Geometry: final body of the model. Coordinates: model frame, mm. Give positions to 0.01 mm unless a question says otherwise; leave off trailing zeros. Order: outer loops, then holes, each group sorted by start corner. A loop starts at its lowest first (then second) coordinate and runs counter-clockwise, first axis right, second up. Notation, with made-up numbers: (-28, 49.5) - (10, 49.5) arc R6 ccw to (10, 59.5) - close; hole circle Ø7 at (-13.5, 70). An arc over 180 degrees is marked (long way). One line per question, with ' | ' between items. Start each with the question number.
from build123d import *

# Parameters (mm, degrees)
SKETCH2_W               = 80
SKETCH2_H               = 47.65
BOSS_EXTRUDE1_DEPTH     = 3.175
SKETCH3_W               = 15
SKETCH3_H               = 3.5
BOSS_EXTRUDE2_DEPTH     = 3.175
SKETCH4_W               = 3.5
SKETCH4_H               = 15
BOSS_EXTRUDE3_DEPTH     = 3.175
MIRROR2_COPY_1_SKETCH_W = 3.5
MIRROR2_COPY_1_SKETCH_H = 15
MIRROR2_COPY_1_DEPTH    = 3.175
MIRROR2_COPY_2_SKETCH_W = 3.5
MIRROR2_COPY_2_SKETCH_H = 15
MIRROR2_COPY_2_DEPTH    = 3.175
SKETCH5_R               = 2.05
CUT_EXTRUDE1_DEPTH      = 20
SKETCH6_W               = 18
SKETCH6_H               = 30
CUT_EXTRUDE2_DEPTH      = 52.468303353
FILLET1_R               = 2.5
MIRROR4_COPY_1_SKETCH_R = 2.05
MIRROR4_COPY_1_DEPTH    = 20
SKETCH8_R               = 1.5
CUT_EXTRUDE4_DEPTH      = 10
LPATTERN1_COUNT         = 3
LPATTERN1_PITCH         = 12.8
MIRROR5_COPY_1_SKETCH_R = 1.5
MIRROR5_COPY_1_DEPTH    = 10
MIRROR5_COPY_2_SKETCH_R = 1.5
MIRROR5_COPY_2_DEPTH    = 10
SKETCH9_W               = 10
SKETCH9_H               = 3.5
BOSS_EXTRUDE4_DEPTH     = 3.175


with BuildPart() as part:
    # Sketch2 → Boss-Extrude1 (new body)
    with BuildSketch(Plane(origin=(0, 0, 0), x_dir=(1, 0, 0), z_dir=(0, 1, 0))):
        Rectangle(SKETCH2_W, SKETCH2_H)
    extrude(amount=BOSS_EXTRUDE1_DEPTH)

    # Sketch3 → Boss-Extrude2 (add)
    with BuildSketch(Plane(origin=(0, 3.175, 0), x_dir=(1, 0, 0), z_dir=(0, 1, 0))):
        with Locations((0, 25.575)):
            Rectangle(SKETCH3_W, SKETCH3_H)
    boss_extrude2 = extrude(amount=-BOSS_EXTRUDE2_DEPTH)

    # Sketch4 → Boss-Extrude3 (add)
    with BuildSketch(Plane(origin=(0, 3.175, 0), x_dir=(1, 0, 0), z_dir=(0, 1, 0))):
        with Locations((-41.75, 0)):
            Rectangle(SKETCH4_W, SKETCH4_H)
    boss_extrude3 = extrude(amount=-BOSS_EXTRUDE3_DEPTH)

    # Mirror1: Boss-Extrude3 across plane
    add(boss_extrude3.mirror(Plane(origin=(0, 0, 0), x_dir=(0, 0, 1), z_dir=(1, 0, 0))))

    # Mirror2: Boss-Extrude2 across plane
    add(boss_extrude2.mirror(Plane.XY))

    # Mirror2 copy 1 sketch → Mirror2 copy 1 (add)
    with BuildSketch(Plane(origin=(0, 3.175, 0), x_dir=(-1, 0, 0), z_dir=(0, 1, 0))):
        with Locations((-41.75, 0)):
            Rectangle(MIRROR2_COPY_1_SKETCH_W, MIRROR2_COPY_1_SKETCH_H)
    extrude(amount=-MIRROR2_COPY_1_DEPTH)

    # Mirror2 copy 2 sketch → Mirror2 copy 2 (add)
    with BuildSketch(Plane(origin=(0, 3.175, 0), x_dir=(1, 0, 0), z_dir=(0, 1, 0))):
        with Locations((-41.75, 0)):
            Rectangle(MIRROR2_COPY_2_SKETCH_W, MIRROR2_COPY_2_SKETCH_H)
    extrude(amount=-MIRROR2_COPY_2_DEPTH)

    # Sketch5 → Cut-Extrude1 (cut)
    with BuildSketch(Plane(origin=(0, 3.175, 0), x_dir=(1, 0, 0), z_dir=(0, 1, 0))):
        with Locations(Location((-35, 18.825, 0), (0, 0, 270))):
            Circle(SKETCH5_R)
    cut_extrude1 = extrude(amount=-CUT_EXTRUDE1_DEPTH, mode=Mode.SUBTRACT)

    # Sketch6 → Cut-Extrude2 (cut, through all)
    with BuildSketch(Plane(origin=(0, 3.175, 0), x_dir=(1, 0, 0), z_dir=(0, 1, 0))):
        with Locations((19, 0)):
            Rectangle(SKETCH6_W, SKETCH6_H)
    extrude(amount=-CUT_EXTRUDE2_DEPTH, mode=Mode.SUBTRACT)

    # Fillet1
    fillet1_edges = [part.edges().sort_by_distance(p)[0] for p in [
        (10, 1.5875, 15),
        (10, 1.5875, -15),
        (28, 1.5875, -15),
        (28, 1.5875, 15),
    ]]
    fillet(fillet1_edges, radius=FILLET1_R)

    # Mirror3: Cut-Extrude1 across plane
    add(cut_extrude1.mirror(Plane(origin=(0, 0, 0), x_dir=(0, 0, 1), z_dir=(1, 0, 0))), mode=Mode.SUBTRACT)

    # Mirror4: Cut-Extrude1 across plane
    add(cut_extrude1.mirror(Plane.XY), mode=Mode.SUBTRACT)

    # Mirror4 copy 1 sketch → Mirror4 copy 1 (cut)
    with BuildSketch(Plane(origin=(0, 3.175, 0), x_dir=(-1, 0, 0), z_dir=(0, 1, 0))):
        with Locations(Location((-35, 18.825, 0), (0, 0, 270))):
            Circle(MIRROR4_COPY_1_SKETCH_R)
    extrude(amount=-MIRROR4_COPY_1_DEPTH, mode=Mode.SUBTRACT)

    # Sketch8 → Cut-Extrude4 (cut)
    with BuildSketch(Plane(origin=(0, 3.175, 0), x_dir=(1, 0, 0), z_dir=(0, 1, 0))):
        with Locations(Location((-30.2, 7.95, 0), (0, 0, 270))):
            Circle(SKETCH8_R)
    cut_extrude4 = extrude(amount=-CUT_EXTRUDE4_DEPTH, mode=Mode.SUBTRACT)

    # LPattern1: Cut-Extrude4 ×3
    with Locations(*[(i * LPATTERN1_PITCH, 0, 0) for i in range(1, LPATTERN1_COUNT)]):
        add(cut_extrude4, mode=Mode.SUBTRACT)

    # Mirror5: Cut-Extrude4 across plane
    add(cut_extrude4.mirror(Plane.XY), mode=Mode.SUBTRACT)

    # Mirror5 copy 1 sketch → Mirror5 copy 1 (cut)
    with BuildSketch(Plane(origin=(12.8, 3.175, 0), x_dir=(1, 0, 0), z_dir=(0, 1, 0))):
        with Locations((-30.2, -7.95)):
            Circle(MIRROR5_COPY_1_SKETCH_R)
    extrude(amount=-MIRROR5_COPY_1_DEPTH, mode=Mode.SUBTRACT)

    # Mirror5 copy 2 sketch → Mirror5 copy 2 (cut)
    with BuildSketch(Plane(origin=(25.6, 3.175, 0), x_dir=(1, 0, 0), z_dir=(0, 1, 0))):
        with Locations((-30.2, -7.95)):
            Circle(MIRROR5_COPY_2_SKETCH_R)
    extrude(amount=-MIRROR5_COPY_2_DEPTH, mode=Mode.SUBTRACT)

    # Sketch9 → Boss-Extrude4 (add)
    with BuildSketch(Plane(origin=(0, 0, 0), x_dir=(1, 0, 0), z_dir=(0, 1, 0))):
        with Locations((-27, 25.575)):
            Rectangle(SKETCH9_W, SKETCH9_H)
    extrude(amount=BOSS_EXTRUDE4_DEPTH)


solid = part.part
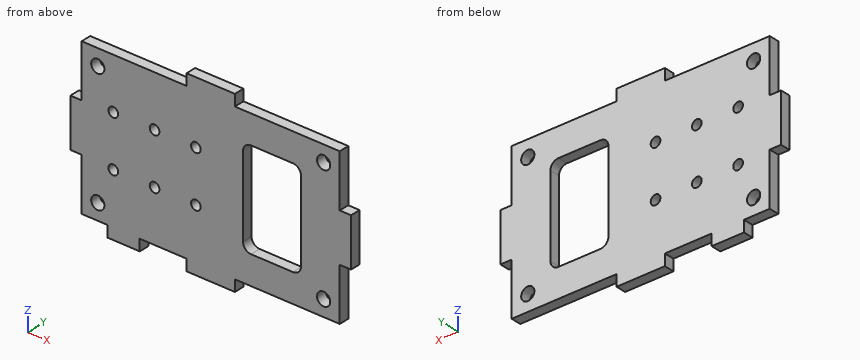
(1) Contact query for flat-ended pins moving along their axis: P1, Ø1.6, axis at x = 17, y = 2, coming from the +Z side (3 decimals); P2, Ø1.6, axis at x = -41.5, y = 1.5, coming from the +Z side; P3, Ø1.6, axis at x = -41.5, y = 1.5, coming from the -Z side. Output: stop coordinate, or through.
(2) Cut plane A-A, the plane z = -11. Return the cut outline in (x, y) (3 decimals), plus the area to 3 significant figures.
(3) Cut plane D-D, the plane x = -4.6. Return the cut outline in (y, z) (3 decimals), plus the area to 3 significant figures.
(4) Cut plane B-B, the plane x = -30.2. Return the cut outline in (y, z) (3 decimals).
(5) Cut plane C-C, the plane z = -4. Return the cut outline in (x, y) (3 decimals), plus the area to 3 significant figures.
(6) Material intervals for line 1 along Z through (x, y) = (35, 1.2) (3 decimals); line 2 along X through (y, z) = (1.15, -7.95); line 3 along Z through (x, y) = (-17.5, 0.5) (3 decimals), sorted ascending. Write a range as from..to.
Results are:
1) P1: z = 23.825 | P2: z = 7.5 | P3: z = -7.5
2) outline: (-40, 0) - (10, 0) - (10, 3.175) - (-40, 3.175) - close; (28, 0) - (40, 0) - (40, 3.175) - (28, 3.175) - close | area: 197 mm2
3) outline: (0, -27.325) - (3.175, -27.325) - (3.175, -9.45) - (0, -9.45) - close; (0, -6.45) - (3.175, -6.45) - (3.175, 6.45) - (0, 6.45) - close; (0, 9.45) - (3.175, 9.45) - (3.175, 27.325) - (0, 27.325) - close | area: 154 mm2
4) outline: (0, -27.325) - (3.175, -27.325) - (3.175, -9.45) - (0, -9.45) - close; (0, -6.45) - (3.175, -6.45) - (3.175, 6.45) - (0, 6.45) - close; (0, 9.45) - (3.175, 9.45) - (3.175, 23.825) - (0, 23.825) - close
5) outline: (-43.5, 0) - (10, 0) - (10, 3.175) - (-43.5, 3.175) - close; (28, 0) - (43.5, 0) - (43.5, 3.175) - (28, 3.175) - close | area: 219 mm2
6) line 1: -23.825..-20.875, -16.775..16.775, 20.875..23.825 | line 2: -40..-31.7, -28.7..-18.9, -15.9..-6.1, -3.1..10, 28..40 | line 3: -23.825..-9.447, -6.453..6.453, 9.447..23.825
